Work out the finished part from the listing and answer in its coordinate system (mm). A direction names the side the tool comes from. Round coordinates to 2 decimals unless told otherwise and drop trailing zeros. Order: outer loops, then holes, each group sorted by start corner. A loop starts at its lowest first (then second) coordinate and runs counter-clockwise, first axis right, second up. Notation, with made-up numbers: M -17,-24 L 2,-24 A17 ccw 2,-7 Z; hole C 8,44.5 d5. An arc over 180 degrees is marked long. Return JSON: item names as keys, results as strings.
from build123d import *

# Parameters (mm, degrees)
ENL_V_MAT_EXTRU_2_DEPTH      = 54.054217551
ENL_V_MAT_EXTRU_2_DEPTH_BACK = 54.054217551
ESQUISSE3_W                  = 6.375
ESQUISSE3_H                  = 4.5
ESQUISSE3_W_2                = 5.625
ESQUISSE3_H_2                = 5.5


with BuildPart() as part:
    # Esquisse1 → Base-R_volution (revolve)
    with BuildSketch(Plane.XY, mode=Mode.PRIVATE) as base_r_volution_sk:
        Polygon((10.75, 49), (10.75, 48), (11.125, 48), (11.125, 18), (9.5, 18), (9.5, 50.5), (11.5, 50.5), (11.5, 49), align=None)
    revolve(base_r_volution_sk.sketch.rotate(Axis((0, 0, 0), (0, 1, 0)), 90), axis=Axis((0, 0, 0), (0, 1, 0)))

    # Esquisse3 → Enl_v. mat.-Extru.2 (cut, two sides: drawn at the far end of the back side and taken through both)
    with BuildSketch(Plane(origin=(0, 0, 0), x_dir=(0, 0, -1), z_dir=(1, 0, 0)).offset(-ENL_V_MAT_EXTRU_2_DEPTH_BACK)):
        with Locations((-7.9375, 31.75)):
            Rectangle(ESQUISSE3_W, ESQUISSE3_H)
        with Locations((8.3125, 28.75)):
            Rectangle(ESQUISSE3_W_2, ESQUISSE3_H_2)
    extrude(amount=ENL_V_MAT_EXTRU_2_DEPTH + ENL_V_MAT_EXTRU_2_DEPTH_BACK, mode=Mode.SUBTRACT)


solid = part.part
Item 1: The mould has two halves that part along X. Classify faces 6 (the cylindrical face through (-0.42, 34.48, 9.49)), 7 (the cylindrical face through (10.86, 32.79, 2.41)), 8 (the flat face through (9, 29, -5.5)): pulls with the +X half, pulls with the -X half, needs draft (parallel to the pull), parting line crosses it, or undercut.
Output:
{"face 6": "undercut", "face 7": "parting line crosses it", "face 8": "needs draft"}
Item 2: Which of the six approach directions +Z, -Z, +X, -X, +Y, -Y give full straight-line access (tool end or side, diameter ignored) to faces 1 (the cylindrical face through (-11.4, 49.7, 1.5)), 2 (the flat face through (-9, 29, -5.5)), 3 (the flat face through (-9, 32, 4.75)), 4 (the flat face through (-9, 50.5, -4)), 5 (the flat face through (8, 49, -8))?
Output:
{"face 1": "+Y, -Y", "face 2": "-Z, +X, -X", "face 3": "+Z, +X, -X", "face 4": "+Z, -Z, +X, -X, +Y", "face 5": "none"}
Item 3: Find section C-C (x = -9). Determine the outline of the cut face in (y, z).
Output:
{"outline": "M 18,-6.54 L 26,-6.54 L 26,-5.5 L 31.5,-5.5 L 31.5,-6.54 L 48,-6.54 L 48,-5.88 L 49,-5.88 L 49,-7.16 L 50.5,-7.16 L 50.5,-3.04 L 18,-3.04 Z; M 18,3.04 L 50.5,3.04 L 50.5,7.16 L 49,7.16 L 49,5.88 L 48,5.88 L 48,6.54 L 34,6.54 L 34,4.75 L 29.5,4.75 L 29.5,6.54 L 18,6.54 Z"}
Item 4: Find section A-A (z = 0). Determine the outline of the cut face in (x, y) (3 decimals), plus the area to 3 significant figures.
Output:
{"outline": "M -11.5,49 L -10.75,49 L -10.75,48 L -11.125,48 L -11.125,18 L -9.5,18 L -9.5,50.5 L -11.5,50.5 Z; M 9.5,18 L 11.125,18 L 11.125,48 L 10.75,48 L 10.75,49 L 11.5,49 L 11.5,50.5 L 9.5,50.5 Z", "area": "106 mm^2"}
Item 5: Find section D-D (y = 37). Determine the outline of the cut face in (x, z) (3 decimals), plus the area to 3 significant figures.
Output:
{"outline": "C 0,0 d22.25; hole C 0,0 d19", "area": "105 mm^2"}
Item 6: Consider line 1 along X through (y, z) = (26.5, 0) (3 decimals); line 2 along Y through (x, z) = (-6.75, 8); line 3 along X through (y, z) = (26, -5). Determine where each line is inside the solid, lowest interval first. Write a range as [from, to].
Output:
{"line 1": "x = [-11.125, -9.5], [9.5, 11.125]", "line 2": "y = [18, 29.5], [34, 50.5]", "line 3": "x = [-9.94, -8.08], [8.08, 9.94]"}
Item 7: Find section B-B (x = 0). Determine the outline of the cut face in (y, z) (3 decimals), plus the area to 4 significant figures.
Output:
{"outline": "M 18,-11.125 L 26,-11.125 L 26,-9.5 L 18,-9.5 Z; M 18,9.5 L 29.5,9.5 L 29.5,11.125 L 18,11.125 Z; M 31.5,-11.125 L 48,-11.125 L 48,-10.75 L 49,-10.75 L 49,-11.5 L 50.5,-11.5 L 50.5,-9.5 L 31.5,-9.5 Z; M 34,9.5 L 50.5,9.5 L 50.5,11.5 L 49,11.5 L 49,10.75 L 48,10.75 L 48,11.125 L 34,11.125 Z", "area": "89.75 mm^2"}
Item 8: Each of these flat-tipped pins is pushed along its axis until it touches: pin 1 (2 mm diameter, centred on y = 42.5, z = 2, fed in from +X); pin 2 (8 mm diameter, centred on x = 3.5, y = 34.5, fed in from +Z) (3 decimals); pin 3 (0.9 mm diameter, centred on x = 9, y = 31.5, fed in from +Z); pin 4 (12 mm diameter, centred on x = -2.5, y = 45, fed in from -Z). Where does it stop, or does it pass through?
Output:
{"pin 1": "stops at x = 11.08", "pin 2": "stops at z = 11.125", "pin 3": "stops at z = 4.75", "pin 4": "stops at z = -11.5"}
